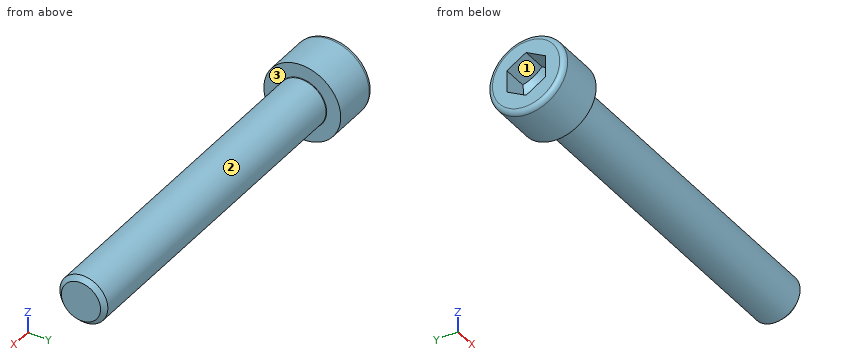
Autodesk Inventor part; units mm, degrees
ref_plane "Work Plane1" through (29, 0, 0) normal (0, -1, 0) x (1, 0, 0)
ref_plane "YZ Plane" through (0, 0, 0) normal (1, 0, 0) x (0, 1, 0)
ref_plane "XZ Plane" through (0, 0, 0) normal (0, 1, 0) x (-1, 0, 0)
sketch "Эскиз1" plane through (0, 0, 0) normal (0, 0, 1) x (1, 0, 0)
  line L0 (-2.3333, 0) -> (70, 0)
  line L1 (70, 0) -> (70, 5)
  line L2 (70, 5) -> (44, 5)
  line L3 (44, 5) -> (43.0797, 5)
  line L4 (43.0797, 5) -> (0, 5)
  line L5 (0, 5) -> (0, 8)
  line L6 (0, 8) -> (-10, 8)
  line L7 (-10, 8) -> (-10, 4.6188)
  line L8 (-10, 4.6188) -> (-5, 4.6188)
  line L9 (-5, 4.6188) -> (-2.3333, 0)
  line L10 (-26, 0) -> (86, 0)
  line L11 (0, -1.6) -> (0, 9.6)
  line L12 (44, 5) -> (0, 5) construction
  dimension "d1" = 26
  dimension "d2" = 0.9203
  dimension "d3" = 10
  dimension "d4" = 5
  dimension "d5" = 60
  dimension "d6" = 10
  dimension "d7" = 10
  dimension "d8" = 9.2376
  dimension "d9" = 16
  dimension "d26" = 70
revolve "Базовый элемент" add sketch "Эскиз1" angle 360 about axis through (-2.3333, 0, 0) along (1, 0, 0)
sketch "Эскиз2" plane through (-10, 0, 0) normal (-1, 0, 0) x (0, 0, 1)
  circle A0 centre (0, 0) radius 4.6188
  line L0 (0, -11.2) -> (0, 11.2)
  line L1 (-11.2, 0) -> (11.2, 0)
  line L2 (4.6188, 0) -> (2.3094, -4)
  line L3 (2.3094, -4) -> (-2.3094, -4)
  line L4 (-2.3094, -4) -> (-4.6188, 0)
  line L5 (-4.6188, 0) -> (-2.3094, 4)
  line L6 (-2.3094, 4) -> (2.3094, 4)
  line L7 (2.3094, 4) -> (4.6188, 0)
extrude "Паз" add sketch "Эскиз2" against normal up to next contours L7 A0 | A0 L2 | L6 L0 A0 | A0 L0 L3 | L0 L6 A0 | A0 L3 L0 | L4 A0 | A0 L5
fillet "Сопряжение1" radius 1 1 edges at (-10, -8, 0)
thread "Резьба"
chamfer "Фаска1" distance 0.9202 distance2 0.9202 1 edges at (70, -5, 0) measured on face at (70, -1.8775, -0.7745)
ref_plane "Work Plane1" through (29, 0, 0) normal (0, -1, 0) x (1, 0, 0)
fillet "Fillet2" radius 0.1 1 edges at (0, -5, 0)
equation "\"d1\" = GEL"
equation "\"d3\" = KOH"
equation "\"d4\" = INTI"
equation "\"d6\" = GD"
equation "\"d7\" = BDM"
equation "\"d8\" = 1.1547 * SW"
equation "\"d9\" = KOD"
equation "\"d30\" = R"
equation "\"d17\" = RR"
equation "\"d13\" = GEL"
equation "\"d15\" = -0.5 * SPD + 0.5 * GD"
equation "\"d16\" = GUL"
equation "\"GD\" = NND"
equation "\"NLG\" = 75"
equation "\"GEL\" = 26"
equation "\"KOD\" = 16"
equation "\"KOH\" = NND"
equation "\"INTI\" = 5"
equation "\"GAL\" = 0.61345 * PTC"
equation "\"GUL\" = 0.61345 * PTC"
equation "\"BDM\" = NND"
equation "\"SW\" = 8"
equation "\"RR\" = 0.1 * NND"
equation "\"SPD\" = NND - 1.2269 * PTC"
equation "\"R\" = 0.1"
equation "\"PHH\" = 0.2"
equation "\"GD1\" = THREADDIA - 1.2269 * PTC"
equation "\"FAWI\" = 45deg"
equation "\"PTC\" = 1.5"
equation "\"KOH1\" = 9"
equation "\"TOA\" = 30deg"
equation "\"E0\" = 1.155 * SW"
properties part number "AS 1420 - 1973 - M10 x 75" material "Сталь, мягкая"
Check sheet for the modelled part. Datum: model origin and axes. Units: mm. Face numbers are marked on the shaded views. Round coordinates to 2 decimals unless told otherwise and drop trailing zeros. Order: outer loops, then holes, each group sorted by start corner. A loop starts at its lowest first (then second) coordinate and runs counter-clockwise, first axis right, second up.
1) Go/stop test with flat-tipped pins: pin 1 Ø5 at (x, y) = (51, 1) entering from -Z; pin 2 Ø1 at (x, z) = (15, 3) entering from -Y; pin 3 Ø1 at (x, z) = (39, -1) entering from +Y. Record where each tip stops, or that it passes through.
2) Mould release check, pull along Y, two halves, no side actions. Record for the marked faces 1, 2 and 3: +Y half, -Y half, draft (parallel to the pull), parting line (faces both ways), or undercut.
3) Section check A-A (x = 6.5). Record the boundary of the cut face in (y, z).
4) Scan lines: line 1 (X direction, y = 5.75, z = -2.75); line 2 (X direction, y = -1.75, z = 2.5); line 3 (Z direction, x = 35, y = 3). Record each from-to range of solid material in increasing order.
Result:
1. pin 1: stops at z = -5
1. pin 2: stops at y = -4.33
1. pin 3: stops at y = 4.97
2. face 1: undercut
2. face 2: parting line
2. face 3: draft
3. outline: circle Ø10 at (0, 0)
4. line 1: x = -10 to 0
4. line 2: x = -4.1 to 70
4. line 3: z = -4 to 4
